Could you check a few things on this model? Use its own coordinates, in mm. Give positions to 0.01 mm unless a question says otherwise; leave off trailing zeros. Loops run counter-clockwise (first coordinate to the right, second up) from the corner with the lowest first, then second, coordinate; pieces in that order, holes last. Notation, with made-up numbers: (-16, 40.25) -> (26, 40.25) arc R20 ccw to (26, 51.25) -> close; hole circle Ø7 at (-34, 10). An arc over 180 degrees is marked (long way). Write each question's results on one line, items separated by ' | '. Start each with the question number.
Q1. If we section it at A-A, the plane x = 0: List the corners of the cut face in (y, z) for me.
Q2. If we section it at D-D, the plane y = -2.75: List the corners of the cut face in (x, z) for me.
Q3. If I drill on line 1 along X through (y, z) = (12.25, 2.6); line 2 along Y through (x, z) = (-11.5, 2.25); line 3 along X through (y, z) = (-4.75, 0.4), over which ranges is the centre line in solid material (lowest first)?
Q4. If we section it at C-C, the plane y = 14.75: List the corners of the cut face in (x, z) for me, plus the area to 3 significant figures.
Q5. If we section it at B-B, the plane x = -6.25: List the corners of the cut face in (y, z) for me.
Q6. Will these pins go through, and if not, where does the flat tip stop? P1, Ø1, axis at y = 1, z = 1.5, coming from the -X side; P2, Ø1, axis at y = 11, z = 1.5, coming from the -X side; P3, Ø2, axis at x = -0.5, z = 2.5, coming from the -Y side.
from build123d import *

# Parameters (mm, degrees)
SKETCH_R           = 3
SKETCH_R_2         = 1.7
PAD_DEPTH          = 3.5
POLARPATTERN_COUNT = 11
POLARPATTERN_ANGLE = 265
PAD001_DEPTH       = 3.5
POCKET_DEPTH       = 0.001
POCKET_DEPTH_BACK  = -3.501


with BuildPart() as part:
    # Sketch → Pad (new body)
    with BuildSketch(Plane.XY):
        with Locations((-8.847328, -8.107082)):
            Circle(SKETCH_R)
        with Locations((-8.847328, -8.107082)):
            Circle(SKETCH_R_2, mode=Mode.SUBTRACT)
    pad = extrude(amount=PAD_DEPTH)

    # PolarPattern: Pad ×11 about axis
    polarpattern_axis = Axis((0, 0, 0), (0, 0, -1))
    for i in range(1, POLARPATTERN_COUNT):
        add(pad.rotate(polarpattern_axis, i * POLARPATTERN_ANGLE / (POLARPATTERN_COUNT - 1)))

    # Sketch001 → Pad001 (join)
    with BuildSketch(Plane.XY):
        with BuildLine():
            ThreePointArc((3, 13.5), (0, 16.5), (-3, 13.5))
            Line((-3, 13.5), (-3, 10.5))
            ThreePointArc((-3, 10.5), (0, 7.5), (3, 10.5))
            Line((3, 13.5), (3, 10.5))
        make_face()
    extrude(amount=PAD001_DEPTH)

    # Sketch002 → Pocket (cut, two sides)
    with BuildSketch(Plane.XY) as pocket_sk:
        with BuildLine():
            ThreePointArc((1.7, 13.6), (0, 15.3), (-1.7, 13.6))
            Line((-1.7, 13.6), (-1.7, 10.4))
            ThreePointArc((-1.7, 10.4), (0, 8.7), (1.7, 10.4))
            Line((1.7, 13.6), (1.7, 10.4))
        make_face()
    extrude(amount=-POCKET_DEPTH, mode=Mode.SUBTRACT)
    extrude(pocket_sk.sketch, amount=-POCKET_DEPTH_BACK, mode=Mode.SUBTRACT)


solid = part.part
Final values:
1) outline: (7.5, 0) -> (8.7, 0) -> (8.7, 3.5) -> (7.5, 3.5) -> close; (15.3, 0) -> (16.5, 0) -> (16.5, 3.5) -> (15.3, 3.5) -> close
2) outline: (-14.48, 0) -> (-13.14, 0) -> (-13.14, 3.5) -> (-14.48, 3.5) -> close; (-9.93, 0) -> (-8.59, 0) -> (-8.59, 3.5) -> (-9.93, 3.5) -> close; (8.59, 0) -> (9.93, 0) -> (9.93, 3.5) -> (8.59, 3.5) -> close; (13.14, 0) -> (14.48, 0) -> (14.48, 3.5) -> (13.14, 3.5) -> close
3) line 1: x = -7.95 to -6.13, -4.57 to -1.7, 1.7 to 4.57, 6.13 to 7.95 | line 2: y = -9.51 to -6.71, -6.31 to -5.01, -1.61 to 0.51, 3.86 to 9.53 | line 3: x = -14.17 to -12.43, -10.64 to -8.9, 8.9 to 10.64, 12.43 to 14.17
4) outline: (-2.73, 0) -> (-1.25, 0) -> (-1.25, 3.5) -> (-2.73, 3.5) -> close; (1.25, 0) -> (2.73, 0) -> (2.73, 3.5) -> (1.25, 3.5) -> close | area: 10.3 mm²
5) outline: (-9.61, 0) -> (-6.61, 0) -> (-6.61, 3.5) -> (-9.61, 3.5) -> close; (7.88, 0) -> (9.29, 0) -> (9.29, 3.5) -> (7.88, 3.5) -> close; (12.18, 0) -> (13.6, 0) -> (13.6, 3.5) -> (12.18, 3.5) -> close
6) P1: stops at x = -14.72 | P2: stops at x = -8.35 | P3: stops at y = 7.5
